Here's how the part is built. I have some questions about the finished solid (model axes, mm). Give positions to 0.01 mm unless a question says otherwise; leave off trailing zeros. Loops run counter-clockwise (first coordinate to the right, second up) from the corner with the lowest first, then second, coordinate; pieces in that order, holes last.
Q1. I need wall thicknesses on probe 1 along X at (y, z) = (12.75, 0) (3 decimals); probe 2 along X at (y, z) = (13.4, 17); probe 3 along X at (y, z) = (12.6, 15.15) (3 decimals). Which ranges of each line are inside material? Lowest first, please.
Q2. Suppose I cut it at B-B (x = 0). List the corners of the cut face in (y, z) for me (3 decimals).
Q3. Suppose I cut it at C-C (z = 15.15). List the corners of the cut face in (x, y) for me (3 decimals).
Q4. Suppose I cut it at A-A (z = 0). List the corners of the cut face in (x, y) for me (3 decimals).
Q5. I'm going to push a flat-ended pin straight in: P1, Ø5.5, axis at x = 16.26, z = 16.26, coming from the +Y side. Where does the tip first touch, or does it pass through?
Q6. Thinking about a two-plate mould opening in X: for faces 1 (the face through (0.077, 13.521, 13.397)), 2 (the face through (19.123, 13.521, 19.061)), 3 (the face through (0, 12, 0)), 4 (the face through (-16.19, 13.52, 14.51)), which applies, pulls with the +X half, pulls with the -X half, needs draft (parallel to the pull), parting line crosses it, or undercut?
Q7. Suppose I cut it at D-D (y = 13.05). Count the separate pieces of the cut face and the enclosed holes in it, and give its area (3 significant figures).
```python
from build123d import *

# Parameters (mm, degrees)
SKETCH1_R               = 11.9
SKETCH1_R_2             = 9.9
BOSS_EXTRUDE3_DEPTH     = 15
SKETCH4_R               = 9.9
BOSS_EXTRUDE4_DEPTH     = 5.1
BOSS_EXTRUDE8_START     = -3
SKETCH12_R              = 19
SKETCH12_R_2            = 11.9
BOSS_EXTRUDE8_DEPTH     = 3
SKETCH14_R              = 1.755
CUT_EXTRUDE4_DEPTH      = 3
CUT_EXTRUDE5_DEPTH      = 25
CUT_EXTRUDE5_DEPTH_BACK = 20
SKETCH15_W              = 38
SKETCH15_H              = 16.079993569
BOSS_EXTRUDE9_START     = -3
SKETCH16_R              = 9.9
BOSS_EXTRUDE9_DEPTH     = 3
BOSS_EXTRUDE10_START    = -3
SKETCH17_W              = 40
SKETCH17_H              = 40
SKETCH17_R              = 19
BOSS_EXTRUDE10_DEPTH    = 3
SKETCH20_W              = 60
SKETCH20_H              = 60
SKETCH20_W_2            = 40
SKETCH20_H_2            = 40
BOSS_EXTRUDE11_DEPTH    = 3
SKETCH21_R              = 1.755
CUT_EXTRUDE7_DEPTH      = 3
SKETCH23_W              = 60
SKETCH23_H              = 60
CUT_EXTRUDE9_DEPTH      = 3


with BuildPart() as part:
    # Sketch1 → Boss-Extrude3 (new body)
    with BuildSketch(Plane(origin=(0, 0, 0), x_dir=(1, 0, 0), z_dir=(0, 1, 0))):
        with Locations(Location((0, 0, 0), (0, 0, 270))):
            Circle(SKETCH1_R)
        with Locations(Location((0, 0, 0), (0, 0, 270))):
            Circle(SKETCH1_R_2, mode=Mode.SUBTRACT)
    extrude(amount=BOSS_EXTRUDE3_DEPTH)

    # Sketch4 → Boss-Extrude4 (add)
    with BuildSketch(Plane.XZ):
        with Locations(Location((0, 0, 0), (0, 0, 270))):
            Circle(SKETCH4_R)
    extrude(amount=-BOSS_EXTRUDE4_DEPTH)

    # Sketch7 → Cut-Revolve2 (revolve, cut)
    with BuildSketch(Plane(origin=(0, 0, 0), x_dir=(0, 0, -1), z_dir=(1, 0, 0))):
        with BuildLine():
            Line((0, 15), (0, -4.8))
            ThreePointArc((0, -4.8), (9.9, 5.1), (0, 15))
        make_face()
    revolve(axis=Axis((0, 15, 0), (0, -1, 0)), mode=Mode.SUBTRACT)

    # Sketch12 → Boss-Extrude8 (add)
    with BuildSketch(Plane(origin=(0, 15, 0), x_dir=(1, 0, 0), z_dir=(0, 1, 0)).offset(BOSS_EXTRUDE8_START)):
        with Locations(Location((0, 0, 0), (0, 0, 270))):
            Circle(SKETCH12_R)
        with Locations(Location((0, 0, 0), (0, 0, 270))):
            Circle(SKETCH12_R_2, mode=Mode.SUBTRACT)
    extrude(amount=BOSS_EXTRUDE8_DEPTH)

    # Sketch14 → Cut-Extrude4 (cut)
    with BuildSketch(Plane(origin=(0, 15, 0), x_dir=(1, 0, 0), z_dir=(0, 1, 0))):
        with Locations(Location((0, 15.15, 0), (0, 0, 270))):
            Circle(SKETCH14_R)
        with Locations(Location((-15.15, 0, 0), (0, 0, 270))):
            Circle(SKETCH14_R)
        with Locations(Location((0, -15.15, 0), (0, 0, 270))):
            Circle(SKETCH14_R)
        with Locations(Location((15.15, 0, 0), (0, 0, 270))):
            Circle(SKETCH14_R)
    extrude(amount=-CUT_EXTRUDE4_DEPTH, mode=Mode.SUBTRACT)

    # Sketch15 → Cut-Extrude5 (cut, two sides: drawn at the far end of the back side and taken through both)
    with BuildSketch(Plane(origin=(0, 0, 0), x_dir=(0, 0, -1), z_dir=(1, 0, 0)).offset(-CUT_EXTRUDE5_DEPTH_BACK)):
        with Locations((0, 3.960003216)):
            Rectangle(SKETCH15_W, SKETCH15_H)
    extrude(amount=CUT_EXTRUDE5_DEPTH + CUT_EXTRUDE5_DEPTH_BACK, mode=Mode.SUBTRACT)

    # Sketch16 → Boss-Extrude9 (add)
    with BuildSketch(Plane(origin=(0, 15, 0), x_dir=(1, 0, 0), z_dir=(0, 1, 0)).offset(BOSS_EXTRUDE9_START)):
        Circle(SKETCH16_R)
    extrude(amount=BOSS_EXTRUDE9_DEPTH)

    # Sketch17 → Boss-Extrude10 (add)
    with BuildSketch(Plane(origin=(0, 15, 0), x_dir=(1, 0, 0), z_dir=(0, 1, 0)).offset(BOSS_EXTRUDE10_START)):
        Rectangle(SKETCH17_W, SKETCH17_H)
        Circle(SKETCH17_R, mode=Mode.SUBTRACT)
    extrude(amount=BOSS_EXTRUDE10_DEPTH)

    # Sketch20 → Boss-Extrude11 (add)
    with BuildSketch(Plane(origin=(0, 15, 0), x_dir=(1, 0, 0), z_dir=(0, 1, 0))):
        Rectangle(SKETCH20_W, SKETCH20_H)
        Rectangle(SKETCH20_W_2, SKETCH20_H_2, mode=Mode.SUBTRACT)
    extrude(amount=-BOSS_EXTRUDE11_DEPTH)

    # Sketch21 → Cut-Extrude7 (cut)
    with BuildSketch(Plane(origin=(0, 15, 0), x_dir=(1, 0, 0), z_dir=(0, 1, 0))):
        with Locations(Location((-16.263455967, 16.263455967, 0), (0, 0, 270))):
            Circle(SKETCH21_R)
        with Locations(Location((-16.263455967, -16.263455967, 0), (0, 0, 270))):
            Circle(SKETCH21_R)
        with Locations(Location((16.263455967, 16.263455967, 0), (0, 0, 270))):
            Circle(SKETCH21_R)
        with Locations(Location((16.263455967, -16.263455967, 0), (0, 0, 270))):
            Circle(SKETCH21_R)
    extrude(amount=-CUT_EXTRUDE7_DEPTH, mode=Mode.SUBTRACT)

    # Sketch23 → Cut-Extrude9 (cut)
    with BuildSketch(Plane(origin=(0, 15, 0), x_dir=(1, 0, 0), z_dir=(0, 1, 0))):
        Rectangle(SKETCH23_W, SKETCH23_H)
        with BuildLine():
            Line((-20.263455967, -16.263455967), (-20.263455967, 16.263455967))
            ThreePointArc((-20.263455967, 16.263455967), (-19.091883092, 19.091883092), (-16.263455967, 20.263455967))
            Line((-16.263455967, 20.263455967), (16.263455967, 20.263455967))
            ThreePointArc((16.263455967, 20.263455967), (19.091883092, 19.091883092), (20.263455967, 16.263455967))
            Line((20.263455967, 16.263455967), (20.263455967, -16.263455967))
            ThreePointArc((20.263455967, -16.263455967), (19.091883092, -19.091883092), (16.263455967, -20.263455967))
            Line((16.263455967, -20.263455967), (-16.263455967, -20.263455967))
            ThreePointArc((-16.263455967, -20.263455967), (-19.091883092, -19.091883092), (-20.263455967, -16.263455967))
        make_face(mode=Mode.SUBTRACT)
    extrude(amount=-CUT_EXTRUDE9_DEPTH, mode=Mode.SUBTRACT)


solid = part.part
```
Solutions:
1. probe 1: x = -20.263 to -16.905, -13.395 to 13.395, 16.905 to 20.263
1. probe 2: x = -20.2 to -17.86, -14.67 to 14.67, 17.86 to 20.2
1. probe 3: x = -20.263 to -17.62, -14.907 to -1.755, 1.755 to 14.907, 17.62 to 20.263
2. outline: (12, -20.263) - (15, -20.263) - (15, -16.905) - (12, -16.905) - close; (12, -13.395) - (15, -13.395) - (15, 13.395) - (12, 13.395) - close; (12, 16.905) - (15, 16.905) - (15, 20.263) - (12, 20.263) - close
3. outline: (-20.263, 12) - (-17.62, 12) - (-17.62, 15) - (-20.263, 15) - close; (-14.907, 12) - (-1.755, 12) - (-1.755, 15) - (-14.907, 15) - close; (1.755, 12) - (14.907, 12) - (14.907, 15) - (1.755, 15) - close; (17.62, 12) - (20.263, 12) - (20.263, 15) - (17.62, 15) - close
4. outline: (-20.263, 12) - (-16.905, 12) - (-16.905, 15) - (-20.263, 15) - close; (-13.395, 12) - (13.395, 12) - (13.395, 15) - (-13.395, 15) - close; (16.905, 12) - (20.263, 12) - (20.263, 15) - (16.905, 15) - close
5. P1: stops at y = 15
6. face 1: undercut
6. face 2: pulls with the +X half
6. face 3: needs draft
6. face 4: undercut
7. separate pieces: 1
7. enclosed holes: 8
7. area: 1,550 mm2
